Here's the drawing with two shaded views (mm, measured from the low corner). I have some questions. Coordinates: 2 decimals unless noted, no trailing zeros. Write each loop counter-clockwise with the first axis right and the second up, starting at its lowest first coordinate (ties: lowest second). Pieces come first, ordered by that corner, then holes. Notation, with made-up numbers: (19.5, 67) - (51.5, 67) arc R24 cw to (51.5, 82) - close; hole circle Ø10 at (22.5, 0.25). An arc over 180 degrees is marked (long way). Answer in a Markdown table with one row per item. Add a question column.
Item 1: I'm going to push flat-ended pins straight in: pin 1 (1.5 mm diameter, centred on x = 15, z = 0.5, fed in from +Y); pin 2 (1 mm diameter, centred on y = 6, z = 3, fed in from +X); pin 3 (0.6 mm diameter, centred on y = 13, z = 1, fed in from +X). Where does each tip first touch, or does it pass through?
Item 2: Imagine slicing it at B-B (y = 19). Please give me the cut outline in (x, z).
Item 3: If I drill on probe 1 along X at (y, z) = (14.82, 2.35); probe 2 along Y at (x, z) = (24.5, 0.4); probe 3 along X at (y, z) = (23.25, 2.45), over which ranges is the centre line in solid material (lowest first)? Write a range as from..to.
Item 4: Imagine slicing it at A-A (x = 45). Please give me the cut outline in (y, z), plus the area to 3 significant figures.
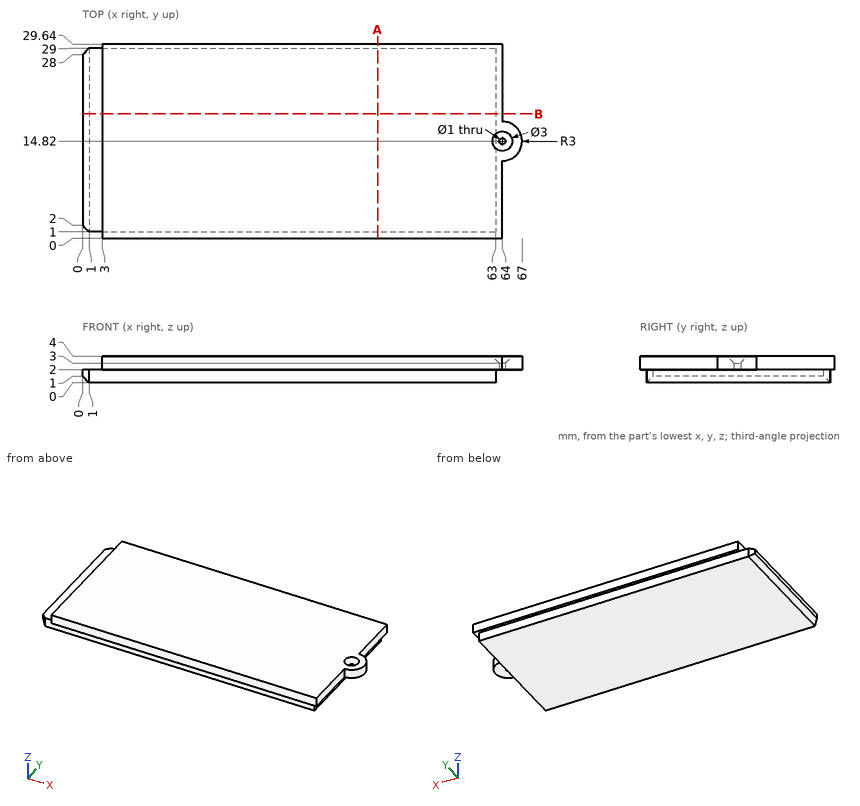
Here are the results:
| question | item | result |
|---|---|---|
| 1 | pin 1 | stops at y = 29 |
| 1 | pin 2 | stops at x = 64 |
| 1 | pin 3 | stops at x = 63 |
| 2 | outline | (0, 1) - (1, 0) - (63, 0) - (63, 2) - (64, 2) - (64, 4) - (3, 4) - (3, 2) - (0, 2) - close |
| 3 | probe 1 | x = 3..63.5, 64.5..67 |
| 3 | probe 2 | y = 1..29 |
| 3 | probe 3 | x = 3..64 |
| 4 | outline | (0, 2) - (1, 2) - (1, 0) - (29, 0) - (29, 2) - (29.64, 2) - (29.64, 4) - (0, 4) - close |
| 4 | area | 115 mm2 |
